from build123d import *

# Parameters (mm, degrees)
F0_W     = 15
F0_H     = 60
F1_DEPTH = 5
F2_W     = 60
F2_H     = 15
F3_DEPTH = 5
F4_W     = 60
F4_H     = 3.95
F5_DEPTH = 10
F6_R     = 1.5
F7_DEPTH = 25
F9_DEPTH = 25
F10_R    = 2.5


with BuildPart() as f1:
    # F0 (on Top) → F1 (new body)
    with BuildSketch(Plane.XY):
        Rectangle(F0_W, F0_H)
    extrude(amount=F1_DEPTH)

    # F2 (on Top) → F3 (join)
    with BuildSketch(Plane.XY):
        with Locations((0, 37.5)):
            Rectangle(F2_W, F2_H)
    extrude(amount=F3_DEPTH)

    # F4 (on face) → F5 (join)
    with BuildSketch(Plane(origin=(0, 0, 0), x_dir=(1, 0, 0), z_dir=(0, 0, -1))):
        with Locations((0, -43.025)):
            Rectangle(F4_W, F4_H)
        with Locations((0, -31.975)):
            Rectangle(F4_W, F4_H)
    extrude(amount=F5_DEPTH)

    # F6 (on face) → F7 (cut)
    with BuildSketch(Plane.XY.offset(5)):
        with Locations((0, -25)):
            Circle(F6_R)
    extrude(amount=-F7_DEPTH, mode=Mode.SUBTRACT)

    # F8 (on face) → F9 (cut)
    with BuildSketch(Plane.XY.offset(5)):
        with BuildLine():
            Line((-1.47942, -12.217379), (-1.47942, -24.752378))
            ThreePointArc((-1.47942, -24.752378), (0, -23.5), (1.47942, -24.752378))
            Line((1.47942, -24.752378), (1.5, -24.752378))
            Line((1.5, -24.752378), (1.5, -14.717379))
            Line((1.5, -14.717379), (7.5, -14.717379))
            Line((7.5, -14.717379), (7.5, -12.217379))
            Line((7.5, -12.217379), (-1.47942, -12.217379))
        make_face()
    extrude(amount=-F9_DEPTH, mode=Mode.SUBTRACT)

    # F10
    f10_edges = [f1.edges().sort_by_distance(p)[0] for p in [
        (-1.47942, -12.217379, 2.5),
    ]]
    fillet(f10_edges, radius=F10_R)


solid = f1.part
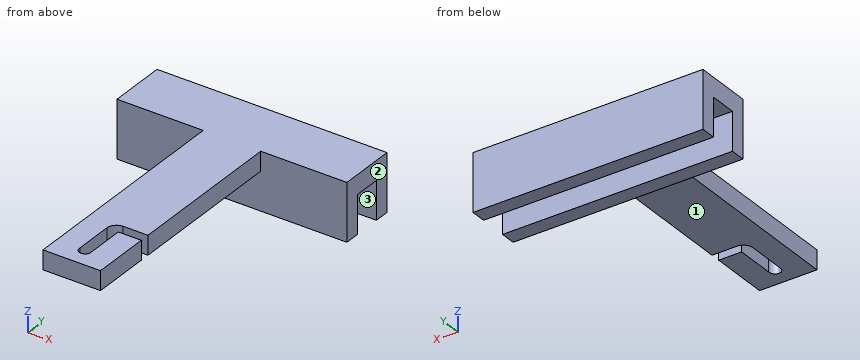
Design review of the part built by this model. Coordinates are the model's own, in mm. Face numbers are marked on the shaded views. A direction names the side the tool comes from. Round coordinates to 2 decimals unless told otherwise and drop trailing zeros. Write each loop counter-clockwise with the first axis right and the second up, starting at its lowest first coordinate (ties: lowest second). Pieces come first, ordered by that corner, then holes. Notation, with made-up numbers: (88, 65.5) - (124, 65.5) arc R32 ccw to (124, 94.5) - close; hole circle Ø3 at (87.25, 30.25). An arc over 180 degrees is marked (long way). Return JSON: item names as keys, results as strings. Group by question number.
Item 1: We need section A-A on z = -1.75. Write out the cut boundary in (x, y).
Item 2: We need section B-B on x = 9. Write out the cut boundary in (y, z).
Item 3: We need section D-D on x = 0. Write out the cut boundary in (y, z).
Item 4: For probe 1 along Y at (x, z) = (20, -4.75); probe 2 along Y at (x, z) = (13, 0.5); probe 3 along Z at (x, y) = (-25, 35.5), list the stretches that pass through material, from the lowest coordinate up. Write a range as [from, to].
Item 5: Machinability: for the marked faces 1, 2 and 3, which of the approach directions +Z, -Z, +X, -X, +Y, -Y give a long, thin tool a straight path to every point of the face, cutting with its end or side? Answer none if there is none.
Item 6: Insertion check: P1, Ø3, axis at x = 7.5, z = -2.5, coming from the -Y side; P2, Ø1.5, axis at y = -18.5, z = 1.5, coming from the +X side; P3, Ø12, axis at x = 0, y = 10, coming from the -Z side. Each pin has a flat end and moves straight along its axis. Give the tip position at first contact, or say it passes through.
Model answer:
{
 "1": {"outline": "(-30, 30) - (30, 30) - (30, 33.95) - (-30, 33.95) - close; (-30, 41.05) - (30, 41.05) - (30, 45) - (-30, 45) - close"},
 "2": {"outline": "(30, -10) - (33.95, -10) - (33.95, 0) - (41.05, 0) - (41.05, -10) - (45, -10) - (45, 5) - (30, 5) - close"},
 "3": {"outline": "(-30, 0) - (-26.5, 0) - (-26.5, 5) - (-30, 5) - close; (-12.44, 0) - (30, 0) - (30, -10) - (33.95, -10) - (33.95, 0) - (41.05, 0) - (41.05, -10) - (45, -10) - (45, 5) - (-12.44, 5) - close"},
 "4": {"probe 1": "y = [30, 33.95], [41.05, 45]", "probe 2": "y = [30, 45]", "probe 3": "z = [0, 5]"},
 "5": {"face 1": "-Z, +X, -X, -Y", "face 2": "+Z, -Z, +X, +Y, -Y", "face 3": "-Z, +X, -X"},
 "6": {"P1": "stops at y = 30", "P2": "stops at x = 7.5", "P3": "stops at z = 0"}
}
